Autodesk Inventor part; units mm, degrees
ref_plane "Plano inicial" through (0, 0, 35) normal (0, 0, 1) x (1, 0, 0)
ref_plane "Plano final" through (0, 0, 965) normal (0, 0, 1) x (1, 0, 0)
ref_plane "Plano de trabajo4" through (0, 29, 965) normal (0, 0, 1) x (1, 0, 0)
ref_plane "Plano inicial" through (0, 0, 35) normal (0, 0, 1) x (1, 0, 0)
ref_plane "Plano final" through (0, 0, 965) normal (0, 0, 1) x (1, 0, 0)
sketch "Boceto" plane through (0, 0, 0) normal (0, 0, 1) x (1, 0, 0)
  line L0 (-25, -21) -> (-25, 21)
  line L1 (-21, 25) -> (21, 25)
  line L2 (25, 21) -> (25, -21)
  line L3 (21, -25) -> (-21, -25)
  arc A0 (-25, -21) -> (-21, -25) centre (-21, -21) ccw
  arc A1 (25, 21) -> (21, 25) centre (21, 21) ccw
  arc A2 (-21, 25) -> (-25, 21) centre (-21, 21) ccw
  arc A3 (21, -25) -> (25, -21) centre (21, -21) ccw
  arc A4 (-21, 23) -> (-23, 21) centre (-21, 21) ccw
  line L4 (-21, 23) -> (21, 23)
  arc A5 (23, 21) -> (21, 23) centre (21, 21) ccw
  line L5 (23, 21) -> (23, -21)
  arc A6 (21, -23) -> (23, -21) centre (21, -21) ccw
  line L6 (21, -23) -> (-21, -23)
  arc A7 (-23, -21) -> (-21, -23) centre (-21, -21) ccw
  line L7 (-23, -21) -> (-23, 21)
  line L8 (0, 36.1598) -> (0, -36.1598) construction
  line L9 (-36.1598, 0) -> (36.1598, 0) construction
  dimension "d7" = 4
  dimension "d9" = 50
  dimension "d11" = 50
  dimension "d12" = 2
  dimension "d15" = 25
  dimension "d16" = 25
extrude "Cuerpo" add sketch "Boceto" along normal up to surface (930 mm away) from surface at 35
sketch "Sketch3" plane through (0, 0, 0) normal (0, 0, 1) x (1, 0, 0)
  line L0 (0, 0) -> (10, 0)
ref_plane "Work Plane3" through (0, 0, 0) normal (0, -1, 0) x (1, 0, 0)
sketch "Sketch4" plane through (0, 0, 0) normal (0, -1, 0) x (1, 0, 0)
  line L0 (-2, 35) -> (12, 35)
  line L1 (-2, 965) -> (12, 965)
  dimension "d18" = 930
ref_plane "Plano de trabajo4" through (0, 29, 965) normal (0, 0, 1) x (1, 0, 0)
split "Dividir1" plane through (0, 29, 965) removes the side toward (0, 0, 1)
ref_plane "Plano de trabajo5" through (0, -29, 35) normal (0, 0, -1) x (-1, 0, 0)
split "Dividir2" plane through (0, -29, 35) removes the side toward (0, 0, -1)
equation "\"d7\" = G_IR"
equation "\"d9\" = G_W"
equation "\"d11\" = G_H"
equation "\"d12\" = G_T"
equation "\"d15\" = 0.5 * d9"
equation "\"d16\" = 0.5 * d11"
equation "\"d3\" = G_L"
equation "\"G_W\" = 50"
equation "\"G_H\" = 50"
equation "\"G_T\" = 2"
equation "\"G_IR\" = 4"
equation "\"G_L\" = d18"
equation "\"G_OFFSET_START\" = -35"
equation "\"G_OFFSET_END\" = 465"
equation "\"d13\" = -G_OFFSET_START"
equation "\"d14\" = G_OFFSET_END + B_L"
properties part number "ISO 10799-2 - 50x50x2 - 930" material "Galvanizado catalogo 1"
CAD build for the part. Positions are in the model's coordinates, mm. A direction names the side the tool comes from. Round coordinates to 2 decimals unless told otherwise and drop trailing zeros. Loops run counter-clockwise (first coordinate to the right, second up) from the corner with the lowest first, then second, coordinate; pieces in that order, holes last. Notation, with made-up numbers: M -13,85.5 L 36,85.5 A23 cw 36,118.5 Z; hole C -27,12.25 d5. An arc over 180 degrees is marked long. One line per question, with ' | ' between items. Start each with the question number.
Item 1: Pin check, flat tip, straight feed: pin 1 Ø5 at (x, y) = (-19, 12) entering from +Z. Stop position of the tip, or through.
Item 2: Two-plate mould, pull along Y, no slides. Class faces 3 (the flat face through (0, 23, 493)), 4 (the flat face through (0, 25, 493)), 5 (the flat face through (-25, 0, 493)), 6 (the flat face through (-23, 0, 493)): pulls with the +Y half, pulls with the -Y half, needs draft (parallel to the pull), parting line crosses it, or undercut.
Item 3: Cut at B-B, the plane z = 597. Write the cut outline in (x, y).
Item 4: Cut at A-A, the plane x = -12.5. Write the cut outline in (y, z).
Item 5: Which spindle directions (+Z, -Z, +X, -X, +Y, -Y) get a long thin tool onto all of the face, cutting with end or side? Do faces 1 (the flat face through (25, 0, 493)), 2 (the flat face through (0, -23, 493)). Say none if no direction does.
Item 6: Wall check: line 1 (Y direction, x = -17, z = 75.5); line 2 (X direction, y = 22, z = 353). Give the ranges that are in metal, low to high.
Responses:
1) pin 1: passes through
2) face 3: undercut | face 4: pulls with the +Y half | face 5: needs draft | face 6: undercut
3) outline: M -25,-21 A4 ccw -21,-25 L 21,-25 A4 ccw 25,-21 L 25,21 A4 ccw 21,25 L -21,25 A4 ccw -25,21 Z; hole M -23,-21 A2 ccw -21,-23 L 21,-23 A2 ccw 23,-21 L 23,21 A2 ccw 21,23 L -21,23 A2 ccw -23,21 Z
4) outline: M -25,35 L -23,35 L -23,965 L -25,965 Z; M 23,35 L 25,35 L 25,965 L 23,965 Z
5) face 1: +Z, -Z, +X, +Y, -Y | face 2: +Z, -Z
6) line 1: y = -25 to -23, 23 to 25 | line 2: x = -24.87 to -22.73, 22.73 to 24.87
